Read the model definition and answer for the solid it produces. Units are mm, in the model's axes. A direction names the side the tool comes from. Give positions to 0.01 mm unless a question says otherwise; leave off trailing zeros.
```python
from build123d import *

# Parameters (mm, degrees)
F1_DEPTH = 6.35
F3_R     = 1.27
F2_R     = 1.27
F4_DEPTH = 5.08


with BuildPart() as f1:
    # F0 (on Top) → F1 (new body)
    with BuildSketch(Plane.XY):
        Polygon((24.178737, 52.94433), (-52.021263, -23.25567), (24.178737, -23.25567), align=None)
        Polygon((17.828737, -16.90567), (5.128737, -16.90567), (17.828737, -4.20567), align=None, mode=Mode.SUBTRACT)
        Polygon((-3.851519, -16.90567), (-36.691007, -16.90567), (17.828737, 37.614073), (17.828737, 4.774586), align=None, mode=Mode.SUBTRACT)
    extrude(amount=F1_DEPTH)

    # F3
    f3_edges = [f1.edges().sort_by_distance(p)[0] for p in [
        (-13.921263, 14.84433, 6.35),
        (-13.921263, -23.25567, 6.35),
        (24.178737, 14.84433, 6.35),
        (11.478737, -16.90567, 6.35),
        (11.478737, -10.55567, 6.35),
        (17.828737, -10.55567, 6.35),
        (17.828737, 21.19433, 6.35),
        (6.988609, -6.065542, 6.35),
        (-20.271263, -16.90567, 6.35),
        (-9.431135, 10.354202, 6.35),
        (-13.921263, -23.25567, 0),
        (-13.921263, 14.84433, 0),
        (24.178737, 14.84433, 0),
        (11.478737, -16.90567, 0),
        (11.478737, -10.55567, 0),
        (17.828737, -10.55567, 0),
        (17.828737, 21.19433, 0),
        (6.988609, -6.065542, 0),
        (-20.271263, -16.90567, 0),
        (-9.431135, 10.354202, 0),
    ]]
    fillet(f3_edges, radius=F3_R)

    # F2 (on face) → F4 (cut)
    with BuildSketch(Plane.XZ.offset(23.25567)):
        with Locations((-13.921263, 3.175)):
            Circle(F2_R)
    extrude(amount=-F4_DEPTH, mode=Mode.SUBTRACT)


solid = f1.part
```
1) Given pin 1 (1.9 mm diameter, centred on y = 17.5, z = 3.5, fed in from -X); pin 2 (1 mm diameter, centred on x = -16, z = 3.5, fed in from +Y); pin 3 (3.5 mm diameter, centred on x = -13.92, z = 3.18, fed in from +Y), each flat-ended and moving along its own axis, determine where each tip first touches the part or whether it passes through.
Final values:
pin 1: stops at x = -12.22
pin 2: stops at y = 13.27
pin 3: stops at y = 16.6
2) A tool of negligible diameter and unlimited length cuts with its end or side. For faces 4 (the face through (11.34, -10.18, 0.38)), 5 (the face through (-14, -18.176, 3)), 6 (the face through (-9.813, 9.973, 3.148)), from which of +Z, -Z, +X, -X, +Y, -Y can it reach the whole face along a straight path? Write none if from no direction.
Final values:
face 4: -Z
face 5: -Y
face 6: +Z, -Z
3) For a pull along Z with two mould halves and no side action, classify faces 1 (the face through (-9.28, 11.02, 0.38)), 2 (the face through (-12.71, -20.75, 3.56)), 3 (the face through (11.39, -10.645, 3.148)) as released by +Z, released by -Z, zero draft, split by the parting line, or undercut.
Final values:
face 1: released by -Z
face 2: undercut
face 3: zero draft
4) Consider L1, parallel to X at y = -15, z = 0.75; L2, parallel to X at y = -15, z = 2; L3, parallel to X at y = 4, z = 1.5. Determine where each line is inside the solid, lowest interval first.
Final values:
L1: x = -43.61 to -34.94, -1.79 to 6.88, 17.94 to 24.07
L2: x = -43.77 to -34.79, -1.95 to 7.03, 17.83 to 24.18
L3: x = -24.77 to -15.79, 17.05 to 24.18
5) The part is cut by section A-A on x = 13.5. Count the separate pieces of the cut face and the enclosed holes in it, and give its area (3 significant figures).
Final values:
separate pieces: 3
enclosed holes: 0
area: 149 mm2
